from build123d import *

# Parameters (mm, degrees)
BOSS_EXTRUDE1_DEPTH = 50
BOSS_EXTRUDE2_DEPTH = 12
BOSS_EXTRUDE3_DEPTH = 5
SKETCH5_W           = 16
SKETCH5_H           = 12
BOSS_EXTRUDE4_DEPTH = 42
SKETCH6_R           = 3
CUT_EXTRUDE1_DEPTH  = 92.449439583
CUT_EXTRUDE2_START  = 14
SKETCH7_R           = 12
CUT_EXTRUDE2_DEPTH  = 74.852148522
SKETCH8_R           = 1.55
CUT_EXTRUDE3_DEPTH  = 92.449439583
SKETCH9_R           = 1.5
CUT_EXTRUDE4_DEPTH  = 42
SKETCH10_R          = 2
CUT_EXTRUDE5_DEPTH  = 10
SKETCH11_R          = 1
CUT_EXTRUDE6_DEPTH  = 92.449439583
SKETCH12_R          = 2
CUT_EXTRUDE7_DEPTH  = 10
SKETCH13_R          = 2
CUT_EXTRUDE8_DEPTH  = 10


with BuildPart() as part:
    # Sketch1 → Boss-Extrude1 (new body)
    with BuildSketch(Plane(origin=(0, 0, 0), x_dir=(0, 0, -1), z_dir=(1, 0, 0))):
        Polygon((-15, 15), (-15, -25), (-10, -20.804501844), (-10, -10), (-10, 10), (10, 10), (10, 15), align=None)
    extrude(amount=BOSS_EXTRUDE1_DEPTH)

    # Sketch2 → Boss-Extrude2 (add)
    with BuildSketch(Plane(origin=(50, 0, 0), x_dir=(0, 0, -1), z_dir=(1, 0, 0))):
        Polygon((-15, 15), (-15, -11.945927107), (-10, -7.750428951), (-10, 10), (10, 10), (10, 15), align=None)
    extrude(amount=BOSS_EXTRUDE2_DEPTH)

    # Sketch4 → Boss-Extrude3 (add)
    with BuildSketch(Plane(origin=(62, 0, 0), x_dir=(0, 0, -1), z_dir=(1, 0, 0))):
        Polygon((10, 15), (-15, 15), (-15, -11.945927107), (-10, -7.750428951), (-10, 10), (10, 10), align=None)
        Polygon((-15, -25), (-10, -20.804501844), (-10, -7.750428951), (-15, -11.945927107), align=None)
    extrude(amount=BOSS_EXTRUDE3_DEPTH)

    # Sketch5 → Boss-Extrude4 (add)
    with BuildSketch(Plane.XY.offset(15)):
        Polygon((67, 15), (0, 15), (0, 10), (46, 10), (62, 10), (67, 10), align=None)
        with Locations((54, 4)):
            Rectangle(SKETCH5_W, SKETCH5_H)
        Polygon((67, -25), (67, 10), (62, 10), (62, -2), (62, -11.945927107), (62, -25), align=None)
    extrude(amount=BOSS_EXTRUDE4_DEPTH)

    # Sketch6 → Cut-Extrude1 (cut, through all)
    with BuildSketch(Plane(origin=(67, 0, 0), x_dir=(0, 0, -1), z_dir=(1, 0, 0))):
        with Locations((-36.15, -11.15)):
            Circle(SKETCH6_R)
    extrude(amount=-CUT_EXTRUDE1_DEPTH, mode=Mode.SUBTRACT)

    # Sketch7 → Cut-Extrude2 (cut, through all)
    with BuildSketch(Plane.ZY.offset(-62).offset(CUT_EXTRUDE2_START)):
        with Locations((36.15, -11.15)):
            Circle(SKETCH7_R)
    extrude(amount=CUT_EXTRUDE2_DEPTH, mode=Mode.SUBTRACT)

    # Sketch8 → Cut-Extrude3 (cut, through all)
    with BuildSketch(Plane(origin=(67, 0, 0), x_dir=(0, 0, -1), z_dir=(1, 0, 0))):
        with Locations((-51.65, 4.35)):
            Circle(SKETCH8_R)
        with Locations((-20.65, 4.35)):
            Circle(SKETCH8_R)
    extrude(amount=-CUT_EXTRUDE3_DEPTH, mode=Mode.SUBTRACT)

    # Sketch9 → Cut-Extrude4 (cut)
    with BuildSketch(Plane(origin=(0, 15, 0), x_dir=(1, 0, 0), z_dir=(0, 1, 0))):
        with Locations(Location((55, -42.5, 0), (0, 0, 270))):
            Circle(SKETCH9_R)
    extrude(amount=-CUT_EXTRUDE4_DEPTH, mode=Mode.SUBTRACT)

    # Sketch10 → Cut-Extrude5 (cut)
    with BuildSketch(Plane(origin=(0, 15, 0), x_dir=(1, 0, 0), z_dir=(0, 1, 0))):
        with Locations(Location((55, -42.5, 0), (0, 0, 270))):
            Circle(SKETCH10_R)
    extrude(amount=-CUT_EXTRUDE5_DEPTH, mode=Mode.SUBTRACT)

    # Sketch11 → Cut-Extrude6 (cut, through all)
    with BuildSketch(Plane(origin=(67, 0, 0), x_dir=(0, 0, -1), z_dir=(1, 0, 0))):
        with Locations((-42.5, 9)):
            Circle(SKETCH11_R)
    extrude(amount=-CUT_EXTRUDE6_DEPTH, mode=Mode.SUBTRACT)

    # Sketch12 → Cut-Extrude7 (cut)
    with BuildSketch(Plane(origin=(0, 15, 0), x_dir=(1, 0, 0), z_dir=(0, 1, 0))):
        with Locations(Location((9.5, 0, 0), (0, 0, 270))):
            Circle(SKETCH12_R)
        with Locations(Location((21.5, 0, 0), (0, 0, 270))):
            Circle(SKETCH12_R)
        with Locations(Location((33.5, 0, 0), (0, 0, 270))):
            Circle(SKETCH12_R)
        with Locations(Location((45.5, 0, 0), (0, 0, 270))):
            Circle(SKETCH12_R)
        with Locations(Location((57.5, 0, 0), (0, 0, 270))):
            Circle(SKETCH12_R)
    extrude(amount=-CUT_EXTRUDE7_DEPTH, mode=Mode.SUBTRACT)

    # Sketch13 → Cut-Extrude8 (cut)
    with BuildSketch(Plane(origin=(0, 0, 10), x_dir=(-1, 0, 0), z_dir=(0, 0, -1))):
        with Locations((-5, 0)):
            Circle(SKETCH13_R)
        with Locations((-16, 0)):
            Circle(SKETCH13_R)
        with Locations((-27, 0)):
            Circle(SKETCH13_R)
    extrude(amount=-CUT_EXTRUDE8_DEPTH, mode=Mode.SUBTRACT)


solid = part.part
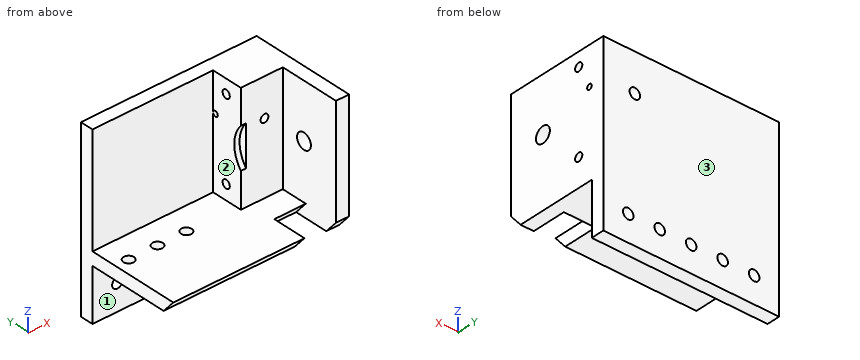
Read the model definition and answer for the solid it produces. Units are mm, in the model's axes. Face numbers are marked on the shaded views. A direction names the side the tool comes from. Round coordinates to 2 decimals unless told otherwise and drop trailing zeros. Write each loop counter-clockwise with the first axis right and the second up, starting at its lowest first coordinate (ties: lowest second). Pieces come first, ordered by that corner, then holes. Notation, with made-up numbers: (-36, 46.25) - (-18, 46.25) arc R13 ccw to (-18, 56.25) - close; hole circle Ø1 at (38.25, -38.75). An arc over 180 degrees is marked (long way). Use a Markdown table: item, result.
(1) The part is cut by section C-C (y = -16). Write down the section's boundary in (x, z).
Reported:
| item | result |
|---|---|
| outline | (0, 10) - (50, 10) - (50, 15) - (0, 15) - close; (62, 10) - (67, 10) - (67, 57) - (62, 57) - close |
(2) Each of these flat-tipped pins is pushed along its axis until it touches: pin 1 Ø11.5 at (y, z) = (-15, 38) entering from -X; pin 2 Ø3 at (x, y) = (41.5, -7) entering from +Z; pin 3 Ø1.8 at (y, z) = (9, 42.5) entering from +X; pin 4 Ø1 at (x, z) = (28.5, 22) entering from -Y. Where does it stop, or does it pass through?
Reported:
| item | result |
|---|---|
| pin 1 | x = 62 |
| pin 2 | z = 15 |
| pin 3 | through |
| pin 4 | y = 10 |
(3) The part is cut by section A-A (z = 0). Write down the section's boundary in (x, y).
Reported:
| item | result |
|---|---|
| outline | (0, 10) - (7.5, 10) - (7.5, 15) - (0, 15) - close; (11.5, 10) - (19.5, 10) - (19.5, 15) - (11.5, 15) - close; (23.5, 10) - (31.5, 10) - (31.5, 15) - (23.5, 15) - close; (35.5, 10) - (43.5, 10) - (43.5, 15) - (35.5, 15) - close; (47.5, 10) - (55.5, 10) - (55.5, 15) - (47.5, 15) - close; (59.5, 10) - (67, 10) - (67, 15) - (59.5, 15) - close |
(4) The part is cut by section D-D (z = 51.65). Write down the section's boundary in (x, y).
Reported:
| item | result |
|---|---|
| outline | (0, 10) - (46, 10) - (46, 5.9) - (67, 5.9) - (67, 15) - (0, 15) - close; (46, -2) - (62, -2) - (62, -25) - (67, -25) - (67, 2.8) - (46, 2.8) - close |
(5) Straight lines are drawn through the part: line 1 along X through (y, z) = (0.25, 42.5); line 2 along Z through (x, y) = (49, 9); line 3 along Y through (x, z) = (60, 42.5). For each, find the intervals that lie inside material, in ascending order. Write a range as [from, to].
Reported:
| item | result |
|---|---|
| line 1 | [46, 53.5], [56.5, 67] |
| line 2 | [10, 41.5], [43.5, 57] |
| line 3 | [-2, 8], [10, 15] |
(6) The part is cut by section B-B (x = 27). Write down the section's boundary in (y, z), then the cut area to 3 significant figures.
Reported:
| item | result |
|---|---|
| outline | (-25, 15) - (-20.8, 10) - (-2, 10) - (-2, 15) - close; (2, 10) - (10, 10) - (10, -10) - (15, -10) - (15, 57) - (10, 57) - (10, 15) - (2, 15) - close |
| area | 480 mm2 |
(7) Which of the six approach directions +Z, -Z, +X, -X, +Y, -Y give full straight-line access (tool end or side, diameter ignored) to the marked faces 1, 2 and 3?
Reported:
| item | result |
|---|---|
| face 1 | -Z, +X, -X, -Y |
| face 2 | +Z, -X, -Y |
| face 3 | +Z, -Z, +X, -X, +Y |
